from build123d import *

# Parameters (mm, degrees)
SKETCH2_W           = 30
SKETCH2_H           = 30
SKETCH3_R           = 13.5
BOSS_EXTRUDE1_DEPTH = 40
BOSS_EXTRUDE2_DEPTH = 30
BOSS_EXTRUDE3_START = -15
BOSS_EXTRUDE3_DEPTH = 30
SKETCH6_R           = 5
BOSS_EXTRUDE4_DEPTH = 43.044915


with BuildPart() as part:
    # Sweep1: sweep along a path in Sketch1
    with BuildLine(Plane(origin=(0, 0, 0), x_dir=(0, 0, -1), z_dir=(1, 0, 0))) as sweep1_path:
        Line((0, 0), (0, 30))
        ThreePointArc((0, 30), (35.147186258, 114.852813742), (120, 150))
    # Sketch2 → Sweep1 (sweep)
    with BuildSketch(Plane(origin=(0, 0, 0), x_dir=(1, 0, 0), z_dir=(0, 1, 0))):
        Rectangle(SKETCH2_W, SKETCH2_H)
    sweep(path=sweep1_path.line)

    # Sketch3 → Boss-Extrude1 (add)
    with BuildSketch(Plane.XZ):
        Circle(SKETCH3_R)
    extrude(amount=BOSS_EXTRUDE1_DEPTH)

    # Sketch4 → Boss-Extrude2 (add)
    with BuildSketch(Plane(origin=(15, 0, 0), x_dir=(0, 0, -1), z_dir=(1, 0, 0))):
        with BuildLine():
            Line((120, 165), (120, 135))
            ThreePointArc((120, 135), (135, 150), (120, 165))
        make_face()
    extrude(amount=-BOSS_EXTRUDE2_DEPTH)

    # Sketch5 → Boss-Extrude3 (add)
    with BuildSketch(Plane(origin=(0, 0, 0), x_dir=(0, 0, -1), z_dir=(1, 0, 0)).offset(BOSS_EXTRUDE3_START)):
        with BuildLine():
            Line((19.707410468, 120.368116529), (11.04715643, 125.368116529))
            Line((11.04715643, 125.368116529), (-6.858503806, 76.172719349))
            ThreePointArc((-6.858503806, 76.172719349), (4.294714537, 99.550606869), (19.707410468, 120.368116529))
        make_face()
    extrude(amount=BOSS_EXTRUDE3_DEPTH)

    # Sketch6 → Boss-Extrude4 (add)
    with BuildSketch(Plane(origin=(0, 98.809646451, -57.047775977), x_dir=(1, 0, 0), z_dir=(0, 0.866025404, -0.5))):
        with Locations((0, -48.116940156)):
            Circle(SKETCH6_R)
    extrude(amount=BOSS_EXTRUDE4_DEPTH)


solid = part.part
Geometry check sheet. Reference: the model listing, model coordinates, mm. A direction names the side the tool comes from. Give positions to 0.01 mm unless a question says otherwise; leave off trailing zeros. Loops run counter-clockwise (first coordinate to the right, second up) from the corner with the lowest first, then second, coordinate; pieces in that order, holes last. Notation, with made-up numbers: M 36,-1.5 L 54,-1.5 A5 cw 54,4.5 Z; hole C 33.25,65 d1. An arc over 180 degrees is marked long. Answer as a JSON object with one key per item and string values. Group by question number.
Item 1: Sectioned sample at D-D on x = -2.25. Record the boundary of the cut face in (y, z).
Item 2: Mould release check, pull along Z, two halves, no side actions. Record for faces 1 (the flat face through (9.06, 122.83, -15.44)), 2 (the cylindrical face through (0.21, 53.118, 13.006)), 3 (the flat face through (-15, 101, -37)): pulls with the +Z half, pulls with the -Z half, needs draft (parallel to the pull), parting line crosses it, or undercut.
Item 3: Sectioned sample at C-C on y = 73.5. Record the boundary of the cut face in (x, z).
Item 4: Sectioned sample at A-A on x = 9. Record the boundary of the cut face in (y, z), plus the area to 3 significant figures.
Item 5: Gauge pin test, flat ends, axial feed: pin 1 (15 mm diameter, centred on x = 2, y = 21, fed in from -Z); pin 2 (3 mm diameter, centred on x = 0, z = -65, fed in from +Y); pin 3 (2 mm diameter, centred on x = 11.5, y = 68.5, fed in from -Z). Record the tip position at first contact, or that the pin passes through.
Item 6: Access from +Z, -Z, +X, -X, +Y, -Y to the whole of each face (thin tool, end or side, straight path). Record for faces 4 (the flat face through (-0.07, 160.11, -36.96)), 5 (the cylindrical face through (-2.93, -19.72, -13.18)), 6 (the flat face through (0, 15, -15)).
Item 7: Sectioned sample at B-B on z = 0. Record the boundary of the cut face in (x, y), plus the area to 3 significant figures.
Item 8: Material ranges on L1, parallel to Z at x = 5, y = 2.5; L2, parallel to Y at x = -11.75, z = -117.5; L3, parallel to Y at x = -5.25, z = -88 (3 decimals), recorded low to high.
Findings below:
{
 "1": {"outline": "M -40,-13.31 L 0,-13.31 L 0,-15 L 30,-15 A105 cw 135,-120 A15 ccw 165,-120 A135 ccw 120.37,-19.71 L 120.64,-19.24 L 157.91,-40.77 L 162.38,-33.03 L 125.1,-11.51 L 125.37,-11.05 L 76.17,6.86 A135 ccw 30,15 L 0,15 L 0,13.31 L -40,13.31 Z"},
 "2": {"face 1": "undercut", "face 2": "pulls with the +Z half", "face 3": "needs draft"},
 "3": {"outline": "M -15,-24.43 L 15,-24.43 L 15,7.8 L -15,7.8 Z"},
 "4": {"outline": "M -40,-10.06 L 0,-10.06 L 0,-15 L 30,-15 A105 cw 135,-120 A15 ccw 165,-120 A135 ccw 120.37,-19.71 L 125.37,-11.05 L 76.17,6.86 A135 ccw 30,15 L 0,15 L 0,10.06 L -40,10.06 Z", "area": "7,890 mm2"},
 "5": {"pin 1": "z = -15", "pin 2": "y = 153.95", "pin 3": "z = -22.71"},
 "6": {"face 4": "+X, -X, +Y", "face 5": "-Y", "face 6": "-Z, +X, -X, -Y"},
 "7": {"outline": "M -15,0 L -13.5,0 L -13.5,-40 L 13.5,-40 L 13.5,0 L 15,0 L 15,95.02 L -15,95.02 Z", "area": "3,930 mm2"},
 "8": {"L1": "-15 to 15", "L2": "134.97 to 164.98", "L3": "130.005 to 161.153"}
}
